Build history of the part. All positions in model axes, mm. Face numbers are marked on the shaded views. A direction names the side the tool comes from. Give positions to 0.01 mm unless a question says otherwise; leave off trailing zeros. Order: outer loops, then holes, each group sorted by start corner. A loop starts at its lowest first (then second) coordinate and runs counter-clockwise, first axis right, second up. Notation, with made-up numbers: M 46.5,-33.5 L 69.5,-33.5 A21 cw 69.5,-9.5 Z; hole C -10,-1.5 d8. An arc over 180 degrees is marked long. Use CSV: the item, a comma, the result in double quotes. Start each with the question number.
Item 1: Band-saw the part on B-B on y = 0. Write the cut outline in (x, z).
Item 2: Pin check, flat tip, straight feed: P1, Ø4.5, axis at x = -1.5, y = 13, coming from the -Z side. Stop position of the tip, or through.
Item 3: Band-saw the part on A-A on x = 0. Write the cut outline in (y, z), plus the area to 3 significant figures.
Item 4: Wall check: line 1 along Y through (x, z) = (0, 4.75); line 2 along Z through (x, y) = (4, 17); line 3 along X through (y, z) = (13, 1). Give the ranges that are in metal, low to high.
Item 5: Band-saw the part on D-D on y = 12. Write the cut outline in (x, z), plus the area to 3 significant figures.
Item 6: Band-saw the part on C-C on z = 2.5. Write the cut outline in (x, y).
Item 7: Which spindle directions (+Z, -Z, +X, -X, +Y, -Y) get a long thin tool onto all of the face, cutting with end or side? Do the marked faces 1 and 2. Say none if no direction does.
Item 8: Two-plate mould, pull along Y, no slides. Class the marked faces 3, 4 and 5: pulls with the +Y half, pulls with the -Y half, needs draft (parallel to the pull), parting line crosses it, or undercut.
Autodesk Inventor part; units mm, degrees
ref_plane "YZ Plane" through (0, 0, 0) normal (1, 0, 0) x (0, 1, 0)
ref_plane "XZ Plane" through (0, 0, 0) normal (0, 1, 0) x (-1, 0, 0)
sketch "Sketch3" plane through (0, 0, 0) normal (0, 0, 1) x (1, 0, 0)
  line L0 (-12.7, -19.05) -> (12.7, -19.05)
  line L1 (12.7, -19.05) -> (12.7, 19.05)
  line L2 (12.7, 19.05) -> (-12.7, 19.05)
  line L3 (-12.7, 19.05) -> (-12.7, -19.05)
  line L4 (-12.7, -19.05) -> (12.7, 19.05) construction
  line L5 (12.7, -19.05) -> (-12.7, 19.05) construction
  point P0 (0, 0)
  dimension "d0" = 25.4
  dimension "d1" = 38.1
extrude "Extrusion1" add sketch "Sketch3" along normal mid plane 12.7
sketch "Sketch4" plane through (0, 0, 6.35) normal (0, 0, 1) x (1, 0, 0)
  circle A0 centre (0, 0) radius 2.667
  dimension "d4" = 5.334
extrude "Extrusion2" cut sketch "Sketch4" against normal through all
sketch "Sketch5" plane through (-12.7, -19.05, 6.35) normal (-1, 0, 0) x (0, 0, 1)
  line L0 (3.175, 6.35) -> (50.8, 6.35)
  line L1 (-12.7, 38.1) -> (-12.7, 0)
  line L2 (0, 0) -> (0, 38.1)
  line L3 (-12.7, 0) -> (0, 0)
  line L4 (0, 0) -> (0, 6.35)
  line L5 (0, 6.35) -> (-12.7, 6.35)
  line L6 (-12.7, 6.35) -> (-12.7, 0)
  point P0 (-6.35, 19.05)
  point P1 (-12.7, 6.35)
  dimension "d9" = 6.35
extrude "Extrusion3" cut sketch "Sketch5" against normal through all
sketch "Sketch8" plane through (-12.7, -12.7, -6.35) normal (-1, 0, 0) x (0, 0, 1)
  line L0 (-4.7625, 21.8398) -> (-4.7625, 13.2284)
  line L1 (12.7, 0) -> (12.7, 31.75)
  line L2 (12.7, 0) -> (-4.7625, 0)
  line L3 (-4.7625, 0) -> (-4.7625, 31.75)
  line L4 (-4.7625, 31.75) -> (12.7, 31.75)
  line L5 (12.7, 31.75) -> (12.7, 0)
  point P0 (6.35, 12.7)
  point P1 (-4.7625, 13.2284)
extrude "Extrusion5" add sketch "Sketch8" along normal blind 6.35
mirror "Mirror1" about plane through (0, 0, 0) normal (1, 0, 0) of "Extrusion5"
sketch "Sketch6" plane through (0, 0, 0) normal (0, 0, 1) x (1, 0, 0)
  circle A0 centre (0, 25.4) radius 15.367
  point P0 (0, 0)
  dimension "d10" = 25.4
  dimension "d13" = 30.734
extrude "cutOutForGuide" cut sketch "Sketch6" along normal mid plane 11.0998
sketch "Sketch9" plane through (0, 0, 6.35) normal (0, 0, 1) x (1, 0, 0)
  circle A0 centre (0, 0) radius 3.1242
  dimension "d16" = 6.2484
extrude "Extrusion6" cut sketch "Sketch9" against normal blind 9.525
split "Split1" plane through (0, 0, 0) removes the side toward (0, 0, -1)
properties part number "preventWireJumpingSingleSupportSliceA" material "PBT Plastic"
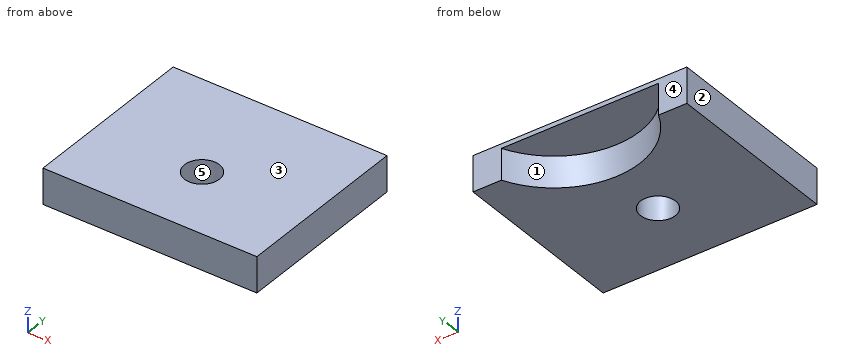
Model answer:
1,outline,"M -19.05,0 L -3.12,0 L -3.12,6.35 L -19.05,6.35 Z; M 3.12,0 L 19.05,0 L 19.05,6.35 L 3.12,6.35 Z"
2,P1,"stops at z = 5.55"
3,outline,"M -12.7,0 L -3.12,0 L -3.12,6.35 L -12.7,6.35 Z; M 3.12,0 L 10.03,0 L 10.03,5.55 L 19.05,5.55 L 19.05,6.35 L 3.12,6.35 Z"
3,area,"112 mm^2"
4,line 1,"y = -12.7 to -3.12, 3.12 to 10.03"
4,line 2,"z = 5.55 to 6.35"
4,line 3,"x = -19.05 to -9.08, 9.08 to 19.05"
5,outline,"M -19.05,0 L -7.52,0 L -7.52,5.55 L 7.52,5.55 L 7.52,0 L 19.05,0 L 19.05,6.35 L -19.05,6.35 Z"
5,area,"158 mm^2"
6,outline,"M -19.05,-12.7 L 19.05,-12.7 L 19.05,19.05 L 13.99,19.05 A15.37 cw -13.99,19.05 L -19.05,19.05 Z; hole C 0,0 d6.25"
7,face 1,"-Z, +Y"
7,face 2,"+Z, -Z, -X, +Y, -Y"
8,face 3,"needs draft"
8,face 4,"pulls with the +Y half"
8,face 5,"undercut"
